Autodesk Inventor part; units mm, degrees
ref_plane "YZ Plane" through (0, 0, 0) normal (1, 0, 0) x (0, 1, 0)
ref_plane "XZ Plane" through (0, 0, 0) normal (0, 1, 0) x (-1, 0, 0)
ref_plane "XY Plane" through (0, 0, 0) normal (0, 0, 1) x (1, 0, 0)
sketch "Sketch1" plane through (0, 0, 0) normal (0, 0, 1) x (1, 0, 0)
  line L0 (-21.05, -12.5) -> (21.05, -12.5)
  line L1 (21.05, -12.5) -> (21.05, 12.5)
  line L2 (21.05, 12.5) -> (-21.05, 12.5)
  line L3 (-21.05, 12.5) -> (-21.05, -12.5)
  line L4 (-21.05, -12.5) -> (21.05, 12.5) construction
  line L5 (21.05, -12.5) -> (-21.05, 12.5) construction
  point P0 (0, 0)
  dimension "d0" = 42.1
  dimension "d1" = 25
extrude "Plate1" add sketch "Sketch1" along normal blind 1.5
sketch "Sketch4" plane through (-21.05, 11, 0) normal (0, 1, 0) x (-1, 0, 0)
  line L0 (-42.1, 0) -> (0, 0)
  line L1 (0, 0) -> (0, 25)
  line L2 (0, 25) -> (-42.1, 25)
  line L3 (-42.1, 25) -> (-42.1, 0)
edge flange "Flange1" height 25 angle 90 thickness 1.5 bend radius 0.31 thickness toward (0, 1, 0) relief tear relief width 1.5 relief depth 0.75 edges at (0, 12.5, 1.5) wall of the first edge with corners at (21.05, 11, 0) (-21.05, 11, 0) (-21.05, 11, 25) (21.05, 11, 25)
bend "Bend1"
corner "Corner1"
sketch "Sketch5" plane through (-21.05, 11, 25) normal (0, -1, 0) x (1, 0, 0)
  circle A0 centre (21.05, -45.25) radius 40
  circle A1 centre (21.05, -45.25) radius 53
  point P0 (21.05, -25)
  dimension "d23" = 13
extrude "Cut1" cut sketch "Sketch5" against normal blind 1.5
fillet "Corner Round1" radius 1 2 edges at (21.05, -12.5, 0.75) (-21.05, -12.5, 0.75)
sketch "Sketch6" plane through (-21.05, 11, 1.81) normal (0, -1, 0) x (1, 0, 0)
  line L0 (0, 0) -> (42.1, 0)
  arc A0 (42.1, 11.9532) -> (0, 11.9532) centre (21.05, -22.06) ccw
  line L1 (21.05, 0) -> (21.05, 17.94) construction
  point P0 (21.05, -1.81)
  point P1 (3.05, 3)
  point P2 (3.05, 10)
  point P3 (21.05, 13)
  point P4 (21.05, 3)
  point P5 (39.05, 3)
  point P6 (39.05, 10)
  dimension "d27" = 10
  dimension "d28" = 3
  dimension "d29" = 18
  dimension "d30" = 7
hole "Hole2" at (-18, 11, 4.81) at (-18, 11, 11.81) at (0, 11, 14.81) at (0, 11, 4.81) at (18, 11, 4.81) at (18, 11, 11.81) direction (0, 1, 0) diameter 2.1 end through all
sketch "Sketch7" plane through (0, 0, 1.5) normal (0, 0, 1) x (1, 0, 0)
  circle A0 centre (17.55, -8.955) radius 0.7835
  circle A1 centre (2.45, -8.955) radius 0.7835
  circle A2 centre (2.45, 6.095) radius 0.7835
  circle A3 centre (17.55, 6.095) radius 0.7835
  circle A4 centre (-17.55, 6.095) radius 0.7835
  circle A5 centre (-17.55, -8.955) radius 0.7835
  point P0 (0, 0)
hole "Hole3" at (17.55, 6.095, 1.5) at (17.55, -8.955, 1.5) at (2.45, -8.955, 1.5) at (2.45, 6.095, 1.5) at (-17.55, 6.095, 1.5) at (-17.55, -8.955, 1.5) direction (0, 0, -1) diameter 2.1 end through all
sketch "Sketch8" plane through (0, 0, 1.5) normal (0, 0, 1) x (1, 0, 0)
  circle A0 centre (-10.05, -1.43) radius 2.925
  circle A1 centre (-10.05, -1.43) radius 6.6
  point P0 (0, 0)
  dimension "d45" = 13.2
extrude "Cut2" cut sketch "Sketch8" against normal blind 1.5 contours A0 | A1
equation "\"d24\" = Thickness"
equation "\"d43\" = Thickness"
equation "\"d46\" = Thickness"
equation "\"d2\" = Thickness"
equation "\"d13\" = BendReliefWidth"
equation "\"d14\" = BendReliefDepth"
equation "\"d15\" = MinimumRemnant"
equation "\"d16\" = TransitionRadius"
equation "\"d19\" = BendRadius"
equation "\"d20\" = CornerReliefSize"
equation "\"d21\" = GapSize"
equation "\"d22\" = JacobiRadiusSize"
equation "\"BendReliefWidth\" = Thickness"
equation "\"BendReliefDepth\" = 0.5 * Thickness"
equation "\"CornerReliefSize\" = 4 * Thickness"
equation "\"MinimumRemnant\" = 2 * Thickness"
equation "\"TransitionRadius\" = BendRadius"
equation "\"JacobiRadiusSize\" = BendRadius"
equation "\"GapSize\" = Thickness"
properties part number "axis_2_bottom_L_frame(bottom)" material "Aluminum 6061-AHC"
Build history of the part. All positions in model axes, mm. A direction names the side the tool comes from. Coordinates: 2 decimals unless noted, no trailing zeros. Order: outer loops, then holes, each group sorted by start corner. A loop starts at its lowest first (then second) coordinate and runs counter-clockwise, first axis right, second up.
Item 1: Saw through at A-A on y = -1.43. List the corners of the cut face in (x, z).
Filled in:
outline: (-21.05, 0) - (-16.65, 0) - (-16.65, 1.5) - (-21.05, 1.5) - close; (-3.45, 0) - (21.05, 0) - (21.05, 1.5) - (-3.45, 1.5) - close
Item 2: Tool access for faces 4 (the cylindrical face through (-16.6, -9.4, 0.7)), 5 (the flat face through (0, 11, 11)): list every direction of +Z, -Z, +X, -X, +Y, -Y with a clear straight run to the whole face (end or side of a thin tool).
Filled in:
face 4: +Z, -Z
face 5: +Z, +X, -X, -Y
Item 3: Mould opens along X. For faces 1 (the cylindrical face through (-16.975, 11.76, 5.038)), 2 (the cylindrical face through (-20.765, -12.199, 0.76)), 3 (the flat face through (0, -12.5, 1)) say: released by +X, released by -X, zero draft, split by the parting line, or undercut.
Filled in:
face 1: undercut
face 2: released by -X
face 3: zero draft
Item 4: Drop flat-ended pins along their axis: pin 1 Ø1.7 at (x, y) = (17.55, 6.095) entering from -Z; pin 2 Ø7 at (x, y) = (7, -3) entering from +Z; pin 3 Ø9 at (x, z) = (-5.5, 13.5) entering from -Y. Give the stop position or say it passes through.
Filled in:
pin 1: passes through
pin 2: stops at z = 1.5
pin 3: stops at y = 11
Item 5: Drill centre lines: L1, parallel to X at y = 12.05, z = 11.81; L2, parallel to Z at x = 18, y = 11.7; L3, parallel to Y at x = -10.05, z = 0.9. Where is each one in solid material? Low to high.
Filled in:
L1: x = -21.05 to -19.05, -16.95 to 16.95, 19.05 to 21.05
L2: z = 0.31 to 3.76, 5.86 to 10.76, 12.86 to 15.47
L3: y = -12.5 to -8.03, 5.17 to 12.25
Item 6: Saw through at B-B on z = 11.81. List the corners of the cut face in (x, y), then the cut area to 4 significant figures.
Filled in:
outline: (-21.05, 11) - (-19.05, 11) - (-19.05, 12.5) - (-21.05, 12.5) - close; (-16.95, 11) - (16.95, 11) - (16.95, 12.5) - (-16.95, 12.5) - close; (19.05, 11) - (21.05, 11) - (21.05, 12.5) - (19.05, 12.5) - close
area: 56.85 mm2
Item 7: Saw through at D-D on z = 15.25. List the corners of the cut face in (x, y), then the cut area to 3 significant figures.
Filled in:
outline: (-18.43, 11) - (-0.95, 11) - (-0.95, 12.5) - (-18.43, 12.5) - close; (0.95, 11) - (18.43, 11) - (18.43, 12.5) - (0.95, 12.5) - close
area: 52.4 mm2
Item 8: Saw through at C-C on x = -17.55. List the corners of the cut face in (y, z) (3 decimals).
Filled in:
outline: (-12.5, 0) - (-10.005, 0) - (-10.005, 1.5) - (-12.5, 1.5) - close; (-7.905, 0) - (5.045, 0) - (5.045, 1.5) - (-7.905, 1.5) - close; (7.145, 0) - (10.69, 0) arc R1.81 ccw to (12.5, 1.81) - (12.5, 3.861) - (11, 3.861) - (11, 1.81) arc R0.31 cw to (10.69, 1.5) - (7.145, 1.5) - close; (11, 5.759) - (12.5, 5.759) - (12.5, 10.861) - (11, 10.861) - close; (11, 12.759) - (12.5, 12.759) - (12.5, 15.694) - (11, 15.694) - close
